Source: CAD feature listing. Evaluate the final solid. Frame: model axes, mm. A direction names the side the tool comes from. Coordinates: 2 decimals unless noted, no trailing zeros. Write item = value, one per line.
from build123d import *

# Parameters (mm, degrees)
F0_W     = 1000
F0_H     = 2000
F1_DEPTH = 50
F2_W     = 50
F2_H     = 1000
F3_DEPTH = 10
F5_DEPTH = 50.001
F6_R     = 25
F8_D     = 17


with BuildPart() as f1:
    # F0 (on Front) → F1 (new body)
    with BuildSketch(Plane.XZ):
        Rectangle(F0_W, F0_H)
    extrude(amount=F1_DEPTH)

    # F2 (on face) → F3 (cut)
    with BuildSketch(Plane.XZ.offset(50)):
        with Locations((-375, -500)):
            Rectangle(F2_W, F2_H)
    extrude(amount=-F3_DEPTH, mode=Mode.SUBTRACT)

    # F4 (on face) → F5 (cut, through all)
    with BuildSketch(Plane.XZ.offset(50)):
        with BuildLine():
            Line((-500, 400), (-500, 0))
            Line((-500, 0), (-400, 0))
            Line((-400, 0), (-350, 0))
            add(Edge.make_bspline(
                [(-350, 400), (-265.8781409264, 399.6310830116), (-243.3533661906, 298.146550271), (-243.3533661906, 102.0078794031), (-265.8781409264, 0), (-350, 0)],
                knots=[0, 0, 0, 0, 0.3135575596, 0.6864424404, 1, 1, 1, 1], degree=3))
            Line((-350, 400), (-500, 400))
        make_face()
    extrude(amount=-F5_DEPTH, mode=Mode.SUBTRACT)

    # F6
    f6_edges = [f1.edges().sort_by_distance(p)[0] for p in [
        (-500, -25, 400),
        (-500, -25, 0),
    ]]
    fillet(f6_edges, radius=F6_R)

    # F8 (through all)
    with Locations(Plane.XZ.offset(40)):
        with Locations((-375, -50), (-375, -150), (-375, -250), (-375, -350), (-375, -450), (-375, -550), (-375, -650), (-375, -750), (-375, -850), (-375, -950)):
            Hole(F8_D / 2)


solid = f1.part
1) Material intervals for probe 1 along X at (y, z) = (-41.5, -426); probe 2 along X at (y, z) = (-15.5, -751.5); probe 3 along Z at (x, y) = (-276, -25.5), sorted ascending. Write a range as [from, to].
Answer block:
probe_1 = [-500, -400], [-350, 500]
probe_2 = [-500, -383.37], [-366.63, 500]
probe_3 = [-1000, 23.62], [376.18, 1000]
2) Reachability of faces 4 (the flat face through (-412, -25, 400)), 5 (the flat face through (-375, -40, -493)), 6 (the flat face through (-500, -25, 708)) from +Z, -Z, +X, -X, +Y, -Y: full face, straight path, thin tool, end or side. Return the list, or none.
Answer block:
face_4 = -X, +Y, -Y
face_5 = -Z, -Y
face_6 = +Z, -Z, -X, +Y, -Y
3) First-contact query: pin 1 Ø13.5 at (x, z) = (-375, -250) entering from +Y; pin 2 Ø22 at (x, z) = (-375, -650) entering from +Y; pin 3 Ø22 at (x, z) = (-375, -350) entering from -Y. Flat tips, straight axial feed; report the tip coordinate or a pass-through.
Answer block:
pin_1 = through
pin_2 = 0
pin_3 = -40
4) Cut plane A-A, the plane y = -21. Give the number of separate pieces and of enclosed holes in the cut face, and give its area (3 significant figures).
Answer block:
separate_pieces = 1
enclosed_holes = 10
area = 1,900,000 mm2
5) Pull-direction query (Z, two-part tool) for faces 1 (the flat face through (-413, -25, 0)), 2 (the flat face through (-451, -50, -493)), 3 (the flat face through (-7, -25, -1000)); classes: +Z half, -Z half, draft (parallel to the pull), parting line (faces both ways), or undercut.
Answer block:
face_1 = undercut
face_2 = draft
face_3 = -Z half
